Geometry: final body of the model. Coordinates: model frame, mm. Round coordinates to 2 decimals unless told otherwise and drop trailing zeros. Write each loop counter-clockwise with the first axis right and the second up, starting at its lowest first coordinate (ties: lowest second). Pieces come first, ordered by that corner, then holes. Notation, with made-up numbers: M 52,22.5 L 73,22.5 A5 cw 73,29.5 Z; hole C -8.75,-14.5 d6. An arc over 180 degrees is marked long. Answer as CSV lines item,"result". Start each with the question number.
Q1. Section query B-B on x = 0. Output: boundary loops of the cut face in (y, z).
Q2. Mould query, pull axis Y, two halves, no side actions, for faces 1 (the cylindrical face through (5.5, -149.9, 1)), 2 (the cylindrical face through (4.694, -129.915, 0.986)), 3 (the flat face through (1, 115, 2)). Classes: pulls with the +Y half, pulls with the -Y half, needs draft (parallel to the pull), parting line crosses it, or undercut.
Q3. Section query C-C on z = 0.8. Output: boundary loops of the cut face in (x, y), and give its area (3 significant figures).
Q4. Ray query, probe 1 along X at (y, z) = (3.5, 1.3); probe 2 along X at (y, z) = (0, 1); probe 3 along Y at (x, z) = (-8, 0.3). Return the intervals inside material, ascending.
Q5. Section query A-A on y = 0. Output: boundary loops of the cut face in (x, z), and give its area (3 significant figures).
```python
from build123d import *

# Parameters (mm, degrees)
ESQUISSE1_R        = 2.5
BOSS_EXTRU_1_DEPTH = 2


with BuildPart() as part:
    # Esquisse1 → Boss.-Extru.1 (new body)
    with BuildSketch(Plane.XY):
        with BuildLine():
            Line((-74.833147735, 130), (74.833147735, 130))
            ThreePointArc((74.833147735, 130), (0, -150), (-74.833147735, 130))
        make_face()
        with Locations((-98.994949366, 98.994949366)):
            Circle(ESQUISSE1_R, mode=Mode.SUBTRACT)
        with Locations((-98.994949366, -98.994949366)):
            Circle(ESQUISSE1_R, mode=Mode.SUBTRACT)
        with Locations((98.994949366, -98.994949366)):
            Circle(ESQUISSE1_R, mode=Mode.SUBTRACT)
        with Locations((98.994949366, 98.994949366)):
            Circle(ESQUISSE1_R, mode=Mode.SUBTRACT)
        with BuildLine():
            Line((-69.282032303, 110), (69.282032303, 110))
            ThreePointArc((69.282032303, 110), (0, -130), (-69.282032303, 110))
        make_face(mode=Mode.SUBTRACT)
    extrude(amount=BOSS_EXTRU_1_DEPTH)


solid = part.part
```
Entries:
1,outline,"M -150,0 L -130,0 L -130,2 L -150,2 Z; M 110,0 L 130,0 L 130,2 L 110,2 Z"
2,face 1,"parting line crosses it"
2,face 2,"undercut"
2,face 3,"needs draft"
3,outline,"M -74.83,130 A150 ccw long 74.83,130 Z; hole C -98.99,-98.99 d5; hole C -98.99,98.99 d5; hole M -69.28,110 A130 ccw long 69.28,110 Z; hole C 98.99,-98.99 d5; hole C 98.99,98.99 d5"
3,area,"17,400 mm^2"
4,probe 1,"x = -149.96 to -129.95, 129.95 to 149.96"
4,probe 2,"x = -150 to -130, 130 to 150"
4,probe 3,"y = -149.79 to -129.75, 110 to 130"
5,outline,"M -150,0 L -130,0 L -130,2 L -150,2 Z; M 130,0 L 150,0 L 150,2 L 130,2 Z"
5,area,"80.0 mm^2"
